Can you work these out from the model? Positions are in its coordinate system, mm. A direction names the side the tool comes from. Coordinates: 2 decimals unless noted, no trailing zeros. Order: outer loops, then holes, each group sorted by start corner. A loop starts at its lowest first (then second) coordinate and runs counter-clockwise, first axis right, second up. Notation, with made-up numbers: M 33.5,40 L 80.5,40 A21 cw 80.5,46 Z; hole C -39.75,68 d10. An arc over 180 degrees is marked long. Answer as CSV lines item,"result". Start each with the question number.
1. If we section it at C-C (y = -5.5): List the corners of the cut face in (x, z) for me.
2. If we mould it in two halves opening along Y, with no side actions, what happens to faces 1 (the face through (-13.644, -14.713, 5.389)), 2 (the face through (0, -20, 10)), 3 (the face through (-12, -10, -0.041))? For each: released by +Y, released by -Y, zero draft, split by the parting line, or undercut.
3. I need wall thicknesses on line 1 along X through (y, z) = (-13, 2.25); line 2 along X through (y, z) = (-15.25, 17.5); line 3 along Z through (x, y) = (11.75, -11.5). Which ranges of each line are inside material? Lowest first, please. Write a range as from..to.
4. If we section it at A-A (z = 2.5): List the corners of the cut face in (x, y) for me, plus the area to 3 significant figures.
5. If we section it at D-D (x = -10): List the corners of the cut face in (y, z) for me (3 decimals).
6. On a 3-axis mill with a long thin cutter (end or side, diameter ignored), from which of +Z, -Z, +X, -X, +Y, -Y can I reach the whole of each face in a straight line? I mean faces 4 (the face through (12.1, -10, 18)), 5 (the face through (-13.64, -14.59, 12.4)), 6 (the face through (10.75, -10, 20)), 7 (the face through (8.43, -9.86, 0.41)). Say none if no direction works.
7. If we section it at B-B (x = 11.75): List the corners of the cut face in (y, z) for me (3 decimals).
8. Will these pins go through, and if not, where does the flat tip stop? pin 1 (10 mm diameter, centred on x = 4.5, y = -14.5, fed in from +Z); pin 2 (8 mm diameter, centred on x = -2.5, y = -6.5, fed in from -Z).
```python
from build123d import *

# Parameters (mm, degrees)
F1_DEPTH = 20
F2_R     = 2.65
F3_DEPTH = 30
F5_DEPTH = 2.75


with BuildPart() as f1:
    # F0 (on Front) → F1 (new body)
    with BuildSketch(Plane.XZ):
        with BuildLine():
            Line((12.1, 16.959205), (-12.1, 16.959205))
            Line((-12.1, 16.959205), (-12.1, 18.709205))
            Line((-12.1, 18.709205), (-10.75, 18.709205))
            Line((-10.75, 18.709205), (-10.75, 20.359205))
            Line((-10.75, 20.359205), (-15, 20.359205))
            Line((-15, 20.359205), (-15, -0.040795))
            Line((-15, -0.040795), (-9.5, -0.040795))
            ThreePointArc((-9.5, -0.040795), (-8.43934, 0.398545), (-8, 1.459205))
            Line((-8, 1.459205), (-8, 3.359205))
            Line((-8, 3.359205), (-11, 6.359205))
            Line((-11, 6.359205), (-8, 9.359205))
            Line((-8, 9.359205), (8, 9.359205))
            Line((8, 9.359205), (11, 6.359205))
            Line((11, 6.359205), (8, 3.359205))
            Line((8, 3.359205), (8, 1.459205))
            ThreePointArc((8, 1.459205), (8.43934, 0.398545), (9.5, -0.040795))
            Line((9.5, -0.040795), (15, -0.040795))
            Line((15, -0.040795), (15, 20.359205))
            Line((15, 20.359205), (10.75, 20.359205))
            Line((10.75, 20.359205), (10.75, 18.709205))
            Line((10.75, 18.709205), (12.1, 18.709205))
            Line((12.1, 18.709205), (12.1, 16.959205))
        make_face()
    extrude(amount=F1_DEPTH)

    # F2 (on face) → F3 (cut)
    with BuildSketch(Plane.YZ.offset(15)):
        with Locations((-12.625, 8.859205)):
            Circle(F2_R)
    extrude(amount=-F3_DEPTH, mode=Mode.SUBTRACT)

    # F4 (on face) → F5 (cut)
    with BuildSketch(Plane(origin=(-15, 0, 0), x_dir=(0, -1, 0), z_dir=(-1, 0, 0))):
        Polygon((16.61254, 11.302466), (12.502844, 13.534147), (8.515304, 11.090886), (8.63746, 6.415944), (12.747156, 4.184264), (16.734696, 6.627525), align=None)
    extrude(amount=-F5_DEPTH, mode=Mode.SUBTRACT)


solid = f1.part
```
Solved:
1,outline,"M -15,-0.04 L -9.5,-0.04 A1.5 ccw -8,1.46 L -8,3.36 L -11,6.36 L -8,9.36 L 8,9.36 L 11,6.36 L 8,3.36 L 8,1.46 A1.5 ccw 9.5,-0.04 L 15,-0.04 L 15,20.36 L 10.75,20.36 L 10.75,18.71 L 12.1,18.71 L 12.1,16.96 L -12.1,16.96 L -12.1,18.71 L -10.75,18.71 L -10.75,20.36 L -15,20.36 Z"
2,face 1,"undercut"
2,face 2,"released by -Y"
2,face 3,"zero draft"
3,line 1,"-15..-8, 8..15"
3,line 2,"-15..-12.1, 12.1..15"
3,line 3,"-0.04..6.46, 11.26..16.96, 18.71..20.36"
4,outline,"M -15,-20 L -8,-20 L -8,0 L -15,0 Z; M 8,-20 L 15,-20 L 15,0 L 8,0 Z"
4,area,"280 mm²"
5,outline,"M -20,-0.041 L 0,-0.041 L 0,5.359 L -20,5.359 Z; M -20,7.359 L -14.81,7.359 A2.65 cw long -10.44,7.359 L 0,7.359 L 0,16.959 L -20,16.959 Z"
6,face 4,"+Y, -Y"
6,face 5,"-X"
6,face 6,"+Z, +Y, -Y"
6,face 7,"-Z, +Y, -Y"
7,outline,"M -20,-0.041 L 0,-0.041 L 0,16.959 L -20,16.959 Z; M -20,18.709 L 0,18.709 L 0,20.359 L -20,20.359 Z; hole C -12.625,8.859 d5.3"
8,pin 1,"z = 16.96"
8,pin 2,"z = 9.36"
